Source: CAD feature listing. Evaluate the final solid. Frame: model axes, mm. Face numbers are marked on the shaded views. A direction names the side the tool comes from. Give positions to 0.01 mm unless a question says otherwise; leave off trailing zeros. Order: outer loops, then holes, each group sorted by start corner. A loop starts at its lowest first (then second) coordinate and runs counter-clockwise, first axis right, second up. Notation, with made-up numbers: (1.25, 2.5) -> (35.25, 2.5) arc R17 ccw to (35.25, 21.5) -> close; hole circle Ø1 at (63, -21). An arc over 180 degrees is marked (long way). Use CSV: the item, a comma, the result in double quotes.
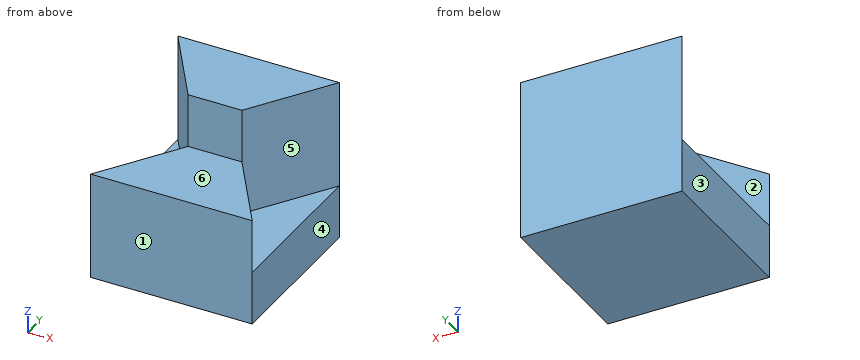
```python
from build123d import *

# Parameters (mm, degrees)
F1_DEPTH = 30
F2_DEPTH = 10
F3_DEPTH = 20


with BuildPart() as f1:
    # F0 (on Top) → F1 (new body)
    with BuildSketch(Plane.XY):
        Polygon((10, 15), (0, 0), (30, 0), (20, 15), align=None)
        Polygon((0, 30), (0, 0), (10, 15), align=None)
        Polygon((20, 15), (30, 0), (30, 30), align=None)
        Polygon((30, 30), (0, 30), (10, 15), (20, 15), align=None)
    extrude(amount=-F1_DEPTH)

    # F0 (on Top) → F2 (cut)
    with BuildSketch(Plane.XY):
        Polygon((10, 15), (0, 0), (30, 0), (20, 15), align=None)
    extrude(amount=-F2_DEPTH, mode=Mode.SUBTRACT)

    # F0 (on Top) → F3 (cut)
    with BuildSketch(Plane.XY):
        Polygon((0, 30), (0, 0), (10, 15), align=None)
        Polygon((20, 15), (30, 0), (30, 30), align=None)
    extrude(amount=-F3_DEPTH, mode=Mode.SUBTRACT)


solid = f1.part
```
1. Access query for the marked faces 4, 5 and 6. Directions: +Z, -Z, +X, -X, +Y, -Y. A direction counts if a zero-diameter tool reaches every point of the face in a straight line with its end or side. Return the directions, or none.
Answer below:
face 4,"+Z, -Z, +X, +Y, -Y"
face 5,"+Z, +X"
face 6,"+Z, +X, -X, -Y"
2. Mould query, pull axis Y, two halves, no side actions, for the marked faces 1, 2 and 3. Classes: released by +Y, released by -Y, zero draft, split by the parting line, or undercut.
Answer below:
face 1,"released by -Y"
face 2,"undercut"
face 3,"zero draft"
3. Section query C-C on z = -14. Return loops of the section in (x, y), plus the area to 3 significant figures.
Answer below:
outline,"(0, 0) -> (30, 0) -> (20, 15) -> (30, 30) -> (0, 30) -> (10, 15) -> close"
area,"600 mm²"
4. Section query D-D on x = 12. Return loops of the section in (y, z).
Answer below:
outline,"(0, -30) -> (30, -30) -> (30, 0) -> (15, 0) -> (15, -10) -> (0, -10) -> close"
5. Section query A-A on y = 19.5. Return loops of the section in (x, z).
Answer below:
outline,"(0, -30) -> (30, -30) -> (30, -20) -> (23, -20) -> (23, 0) -> (7, 0) -> (7, -20) -> (0, -20) -> close"
6. Ray query, line 1 along Y through (x, z) = (20.25, -18.25) (3 decimals); line 2 along Z through (x, y) = (16.5, 9); line 3 along Z through (x, y) = (1.5, 24.5). Return the intervals inside material, ascending.
Answer below:
line 1,"y = 0 to 14.625, 15.375 to 30"
line 2,"z = -30 to -10"
line 3,"z = -30 to -20"
7. Section query B-B on x = 6. Return loops of the section in (y, z), plus the area to 3 significant figures.
Answer below:
outline,"(0, -30) -> (30, -30) -> (30, 0) -> (21, 0) -> (21, -20) -> (9, -20) -> (9, -10) -> (0, -10) -> close"
area,"570 mm²"
8. Pin query (flat end, axial travel): P1, Ø3, axis at x = 5, y = 13, coming from the +Z side; P2, Ø4.5, axis at x = 9.5, y = 8.5, coming from the +Z side; P3, Ø1.5, axis at y = 13.5, z = -18, coming from the -X side. Return the tip coordinate at first contact, or that it passes through.
Answer below:
P1,"stops at z = -20"
P2,"stops at z = -10"
P3,"stops at x = 8.5"
